from build123d import *

# Parameters (mm, degrees)
SKETCH1_W               = 60
SKETCH1_H               = 60
SKETCH1_R               = 3
BOSS_EXTRUDE1_DEPTH     = 5
FILLET1_R               = 6
SKETCH2_R               = 16
SKETCH2_R_2             = 12.75
BOSS_EXTRUDE2_DEPTH     = 15
CUT_EXTRUDE1_DEPTH      = 47.904157598
CUT_EXTRUDE1_DEPTH_BACK = 47.904157598
SKETCH3_R               = 2.5


with BuildPart() as part:
    # Sketch1 → Boss-Extrude1 (new body)
    with BuildSketch(Plane(origin=(0, 0, 0), x_dir=(1, 0, 0), z_dir=(0, 1, 0))):
        Rectangle(SKETCH1_W, SKETCH1_H)
        with Locations(Location((21.5, 21.5, 0), (0, 0, 270))):
            Circle(SKETCH1_R, mode=Mode.SUBTRACT)
        with Locations(Location((-21.5, 21.5, 0), (0, 0, 270))):
            Circle(SKETCH1_R, mode=Mode.SUBTRACT)
        with Locations(Location((-21.5, -21.5, 0), (0, 0, 270))):
            Circle(SKETCH1_R, mode=Mode.SUBTRACT)
        with Locations(Location((21.5, -21.5, 0), (0, 0, 270))):
            Circle(SKETCH1_R, mode=Mode.SUBTRACT)
    extrude(amount=BOSS_EXTRUDE1_DEPTH)

    # Fillet1
    fillet1_edges = [part.edges().sort_by_distance(p)[0] for p in [
        (30, 2.5, 30),
        (-30, 2.5, 30),
        (-30, 2.5, -30),
        (30, 2.5, -30),
    ]]
    fillet(fillet1_edges, radius=FILLET1_R)

    # Sketch2 → Boss-Extrude2 (add)
    with BuildSketch(Plane(origin=(0, 5, 0), x_dir=(1, 0, 0), z_dir=(0, 1, 0))):
        with Locations(Location((0, 0, 0), (0, 0, 90))):
            Circle(SKETCH2_R)
        with Locations(Location((0, 0, 0), (0, 0, 270))):
            Circle(SKETCH2_R_2, mode=Mode.SUBTRACT)
    extrude(amount=BOSS_EXTRUDE2_DEPTH)

    # Sketch3 → Cut-Extrude1 (cut, two sides: drawn at the far end of the back side and taken through both)
    with BuildSketch(Plane(origin=(0, 0, 0), x_dir=(0, 0, -1), z_dir=(1, 0, 0)).offset(-CUT_EXTRUDE1_DEPTH_BACK)):
        with Locations((0, 12.5)):
            Circle(SKETCH3_R)
    extrude(amount=CUT_EXTRUDE1_DEPTH + CUT_EXTRUDE1_DEPTH_BACK, mode=Mode.SUBTRACT)


solid = part.part
The listing builds one solid part. Answer for the finished solid, in the listing's coordinates (mm). A direction names the side the tool comes from. Give positions to 0.01 mm unless a question says otherwise; leave off trailing zeros. Write each loop counter-clockwise with the first axis right and the second up, starting at its lowest first coordinate (ties: lowest second). Pieces come first, ordered by that corner, then holes.
Item 1: Section C-C, the plane y = 3.75 is taken. Write down the section's boundary in (x, z).
Item 2: Determine the mould class of faces 1 (the cylindrical face through (28.196, 2.535, -28.289)), 2 (the cylindrical face through (15.62, 12.4, 3.47)), 3 (the cylindrical face through (-23.3, 2.5, -23.9)), 4 (the flat face through (0, 5, 0)) for opening direction X: released by +X, released by -X, zero draft, split by the parting line, or undercut.
Item 3: Find the intervals of material crossed by line 1 along X through (y, z) = (1.75, 21.5); line 2 along Y through (x, z) = (15.25, 0); line 3 along X through (y, z) = (9, 0), in increasing order.
Item 4: Section D-D, the plane y = 19 is taken. Write down the section's boundary in (x, z).
Item 5: Flat-ended cylindrical pins translate along their axes: P1, Ø20.5, axis at x = 5, z = 1, coming from the +Y side; P2, Ø2, axis at x = -5.5, y = 16, coming from the -Z side; P3, Ø3, axis at y = 12.5, z = 0, coming from the -X side; P4, Ø8, axis at x = -21.5, z = 21.5, coming from the +Y side. Find the tip coordinate at first contact, or state that the pin passes through.
Item 6: Section A-A, the plane x = -21.5 is taken. Write down the section's boundary in (y, z), plus the area to 3 significant figures.
Item 7: Section B-B, the plane z = -21 is taken. Write down the section's boundary in (x, y).
Item 8: Which of the six approach directions +Z, -Z, +X, -X, +Y, -Y give full straight-line access (tool end or side, diameter ignored) to faces 5 (the cylindrical face through (-12.447, 12.395, -2.764)), 6 (the cylindrical face through (-28.289, 2.535, -28.196))?
Completed:
1. outline: (-30, -24) arc R6 ccw to (-24, -30) - (24, -30) arc R6 ccw to (30, -24) - (30, 24) arc R6 ccw to (24, 30) - (-24, 30) arc R6 ccw to (-30, 24) - close; hole circle Ø6 at (-21.5, -21.5); hole circle Ø6 at (-21.5, 21.5); hole circle Ø6 at (21.5, -21.5); hole circle Ø6 at (21.5, 21.5)
2. face 1: released by +X
2. face 2: split by the parting line
2. face 3: undercut
2. face 4: undercut
3. line 1: x = -30 to -24.5, -18.5 to 18.5, 24.5 to 30
3. line 2: y = 0 to 10, 15 to 20
3. line 3: x = -16 to -12.75, 12.75 to 16
4. outline: circle Ø32 at (0, 0); hole circle Ø25.5 at (0, 0)
5. P1: stops at y = 20
5. P2: stops at z = -15.35
5. P3: passes through
5. P4: stops at y = 5
6. outline: (0, -30) - (5, -30) - (5, -24.5) - (0, -24.5) - close; (0, -18.5) - (5, -18.5) - (5, 18.5) - (0, 18.5) - close; (0, 24.5) - (5, 24.5) - (5, 30) - (0, 30) - close
6. area: 240 mm2
7. outline: (-30, 0) - (-24.46, 0) - (-24.46, 5) - (-30, 5) - close; (-18.54, 0) - (18.54, 0) - (18.54, 5) - (-18.54, 5) - close; (24.46, 0) - (30, 0) - (30, 5) - (24.46, 5) - close
8. face 5: +Y
8. face 6: -Z, -X, +Y, -Y
